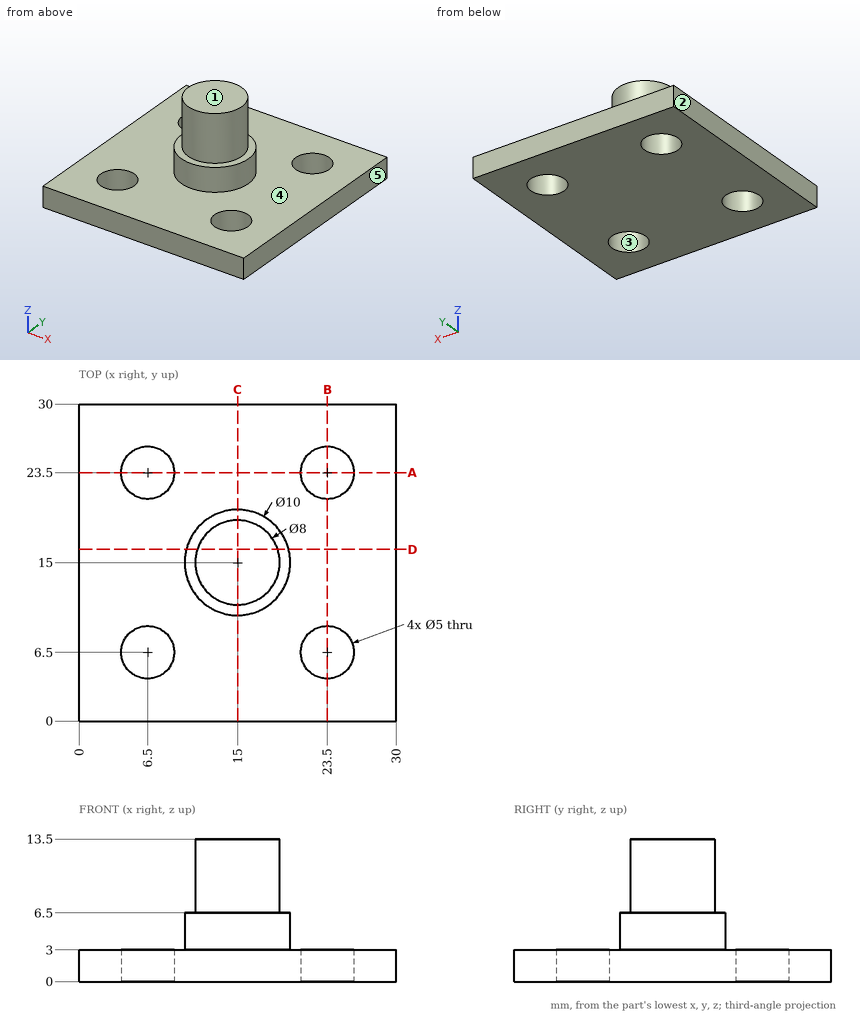
Geometry: see drawing. Coordinates: mm, zero at the bounding-box minimum. A direction names the side the tool comes from. Coordinates: 2 decimals unless noted, no trailing zeros. Loops run counter-clockwise (first coordinate to the right, second up) from the corner with the lowest first, then second, coordinate; pieces in that order, holes last. Notation, with made-up numbers: M -39,-30.75 L -13,-30.75 A29 ccw -13,-6.75 Z; hole C 12.25,-23.5 d4. An arc over 180 degrees is marked long. Put each result on its own line as item: value. Start each with the question number.
1) Cut plane A-A on y = 23.5. Return the cut outline in (x, z), then the cut area to 3 significant figures.
2) Cut plane C-C on x = 15. Return the cut outline in (y, z), then the cut area to 3 significant figures.
3) Cut plane D-D on y = 16.25. Return the cut outline in (x, z), then the cut area to 3 significant figures.
4) Ray query, L1, parallel to Y at x = 6.5, z = 1.9; L2, parallel to Z at x = 13, y = 26.75; L3, parallel to Z at x = 11.75, y = 12. Return the intervals inside material, ascending. Write a range as from..to.
5) Pull-direction query (X, two-part tool) for the marked faces 1, 2 and 3; classes: pulls with the +X half, pulls with the -X half, needs draft (parallel to the pull), parting line crosses it, or undercut.
6) Reachability of the marked faces 4 and 5 from +Z, -Z, +X, -X, +Y, -Y: full face, straight path, thin tool, end or side. Return the list, or none.
7) Contact query for a flat-ended pin moving along its axis: pin 1 Ø3 at (x, y) = (20.5, 7.5) entering from +Z. Output: stop coordinate, or through.
The answers:
1. outline: M 0,0 L 4,0 L 4,3 L 0,3 Z; M 9,0 L 21,0 L 21,3 L 9,3 Z; M 26,0 L 30,0 L 30,3 L 26,3 Z
1. area: 60.0 mm²
2. outline: M 0,0 L 30,0 L 30,3 L 20,3 L 20,6.5 L 19,6.5 L 19,13.5 L 11,13.5 L 11,6.5 L 10,6.5 L 10,3 L 0,3 Z
2. area: 181 mm²
3. outline: M 0,0 L 30,0 L 30,3 L 19.84,3 L 19.84,6.5 L 18.8,6.5 L 18.8,13.5 L 11.2,13.5 L 11.2,6.5 L 10.16,6.5 L 10.16,3 L 0,3 Z
3. area: 177 mm²
4. L1: y = 0..4, 9..21, 26..30
4. L2: z = 0..3
4. L3: z = 0..6.5
5. face 1: needs draft
5. face 2: pulls with the -X half
5. face 3: undercut
6. face 4: +Z
6. face 5: +Z, -Z, +X, +Y, -Y
7. pin 1: stops at z = 3
